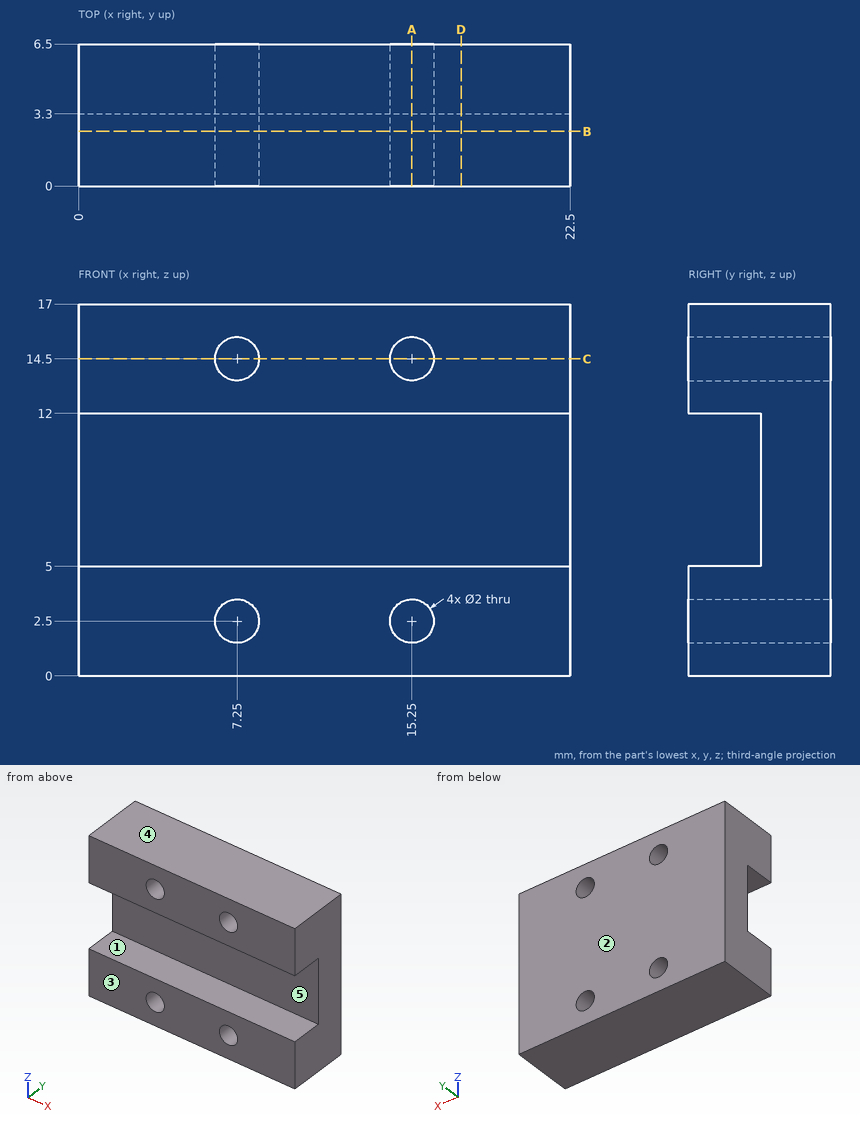
Print and shaded views of the part. All mm, measured from the part's lowest x, y and z. A direction names the side the tool comes from. Give positions to 0.01 mm unless a question says otherwise; leave off trailing zeros. Order: outer loops, then holes, each group sorted by start corner. A loop starts at its lowest first (then second) coordinate and runs counter-clockwise, first axis right, second up. Notation, with made-up numbers: (87, 51.25) - (107, 51.25) arc R9 cw to (107, 55.25) - close; hole circle Ø3 at (-2, 54). An arc over 180 degrees is marked (long way). One line per item, written item: value.
Item 1: Slice it at C-C (z = 14.5). List the corners of the cut face in (x, y).
Response values:
outline: (0, 0) - (6.25, 0) - (6.25, 6.5) - (0, 6.5) - close; (8.25, 0) - (14.25, 0) - (14.25, 6.5) - (8.25, 6.5) - close; (16.25, 0) - (22.5, 0) - (22.5, 6.5) - (16.25, 6.5) - close
Item 2: Pin check, flat tips, straight feed: pin 1 Ø1 at (y, z) = (1.5, 7.5) entering from -X; pin 2 Ø5.5 at (x, z) = (13, 8.5) entering from -Y; pin 3 Ø2.5 at (x, z) = (15.25, 2.5) entering from +Y. Stop position of each tip, or through.
Response values:
pin 1: through
pin 2: y = 3.3
pin 3: y = 6.5
Item 3: Wall check: line 1 (X direction, y = 4.5, z = 2.5); line 2 (Z direction, x = 15.25, y = 4.25); line 3 (Z direction, x = 16.5, y = 1.75). Give the ranges that are in metal, low to high.
Response values:
line 1: 0 to 6.25, 8.25 to 14.25, 16.25 to 22.5
line 2: 0 to 1.5, 3.5 to 13.5, 15.5 to 17
line 3: 0 to 5, 12 to 17
Item 4: Slice it at A-A (x = 15.25). List the corners of the cut face in (y, z).
Response values:
outline: (0, 0) - (6.5, 0) - (6.5, 1.5) - (0, 1.5) - close; (0, 3.5) - (6.5, 3.5) - (6.5, 13.5) - (0, 13.5) - (0, 12) - (3.3, 12) - (3.3, 5) - (0, 5) - close; (0, 15.5) - (6.5, 15.5) - (6.5, 17) - (0, 17) - close
Item 5: Slice it at D-D (x = 17.5). List the corners of the cut face in (y, z), then the cut area to 3 significant figures.
Response values:
outline: (0, 0) - (6.5, 0) - (6.5, 17) - (0, 17) - (0, 12) - (3.3, 12) - (3.3, 5) - (0, 5) - close
area: 87.4 mm2
Item 6: Tool access for the marked faces 1 and 2: list every direction of +Z, -Z, +X, -X, +Y, -Y with a clear straight run to the whole face (end or side of a thin tool).
Response values:
face 1: +X, -X, -Y
face 2: +Z, -Z, +X, -X, +Y
Item 7: Two-plate mould, pull along Z, no slides. Class the marked faces 3, 4 and 5: released by +Z, released by -Z, zero draft, split by the parting line, or undercut.
Response values:
face 3: zero draft
face 4: released by +Z
face 5: undercut
Item 8: Slice it at B-B (y = 2.5). List the corners of the cut face in (x, z).
Response values:
outline: (0, 0) - (22.5, 0) - (22.5, 5) - (0, 5) - close; (0, 12) - (22.5, 12) - (22.5, 17) - (0, 17) - close; hole circle Ø2 at (7.25, 2.5); hole circle Ø2 at (7.25, 14.5); hole circle Ø2 at (15.25, 2.5); hole circle Ø2 at (15.25, 14.5)
